Build history of the part. All positions in model axes, mm. Round coordinates to 2 decimals unless told otherwise and drop trailing zeros. Write each loop counter-clockwise with the first axis right and the second up, starting at its lowest first coordinate (ties: lowest second). Pieces come first, ordered by that corner, then holes. Notation, with made-up numbers: (11, 18.5) -> (55, 18.5) arc R22 ccw to (55, 54.5) -> close; hole circle Ø6 at (13, 1.5). An arc over 180 degrees is marked (long way). Answer in a Markdown table with one row per item. Add a question column.
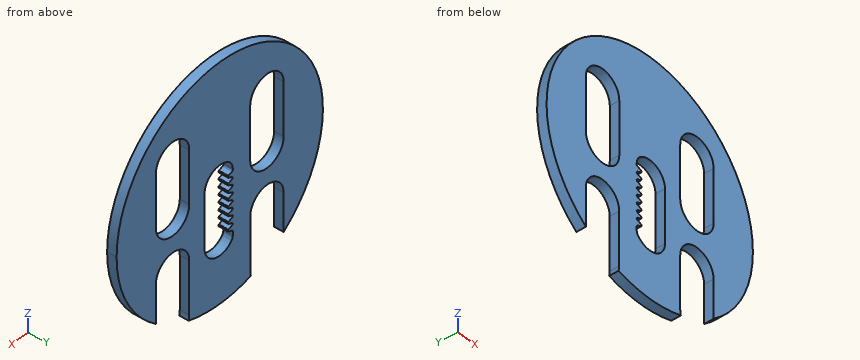
from build123d import *

# Parameters (mm, degrees)
BOSS_EXTRUDE1_DEPTH = 3.175
BOSS_EXTRUDE3_START = -3.175
BOSS_EXTRUDE3_DEPTH = 3.175


# Read off the part's stored shape, not the designer's step: Boss-Extrude3
with BuildPart() as part:
    # Sketch3 → Boss-Extrude1 (new body)
    with BuildSketch(Plane.XZ):
        with BuildLine():
            ThreePointArc((39.2557, 0), (-17.127226966, 35.322345321), (-24.310512242, -30.822215641))
            Line((-24.310512242, -30.822215641), (-24.310512242, -17.960512242))
            ThreePointArc((-24.310512242, -17.960512242), (-17.960512242, -11.610512242), (-11.610512242, -17.960512242))
            Line((-11.610512242, -17.960512242), (-11.610512242, -35.740512242))
            ThreePointArc((-11.610512242, -35.740512242), (-11.667849962, -36.591923676), (-11.838827653, -37.427959366))
            ThreePointArc((-11.838827653, -37.427959366), (0, -39.2557), (11.838827653, -37.427959366))
            ThreePointArc((11.838827653, -37.427959366), (11.667849962, -36.591923676), (11.610512242, -35.740512242))
            Line((11.610512242, -35.740512242), (11.610512242, -17.960512242))
            ThreePointArc((11.610512242, -17.960512242), (17.960512242, -11.610512242), (24.310512242, -17.960512242))
            Line((24.310512242, -17.960512242), (24.310512242, -30.822215641))
            ThreePointArc((24.310512242, -30.822215641), (35.322345321, -17.127226966), (39.2557, 0))
        make_face()
        with BuildLine():
            ThreePointArc((-5.8, 0), (0, 5.8), (5.8, 0))
            Line((5.8, 0), (5.8, -17.78))
            ThreePointArc((5.8, -17.78), (0, -23.58), (-5.8, -17.78))
            Line((-5.8, -17.78), (-5.8, 0))
        make_face(mode=Mode.SUBTRACT)
        with BuildLine():
            ThreePointArc((-11.590512242, 0.180512242), (-17.960512242, -6.189487758), (-24.330512242, 0.180512242))
            Line((-24.330512242, 0.180512242), (-24.330512242, 17.960512242))
            ThreePointArc((-24.330512242, 17.960512242), (-17.960512242, 24.330512242), (-11.590512242, 17.960512242))
            Line((-11.590512242, 17.960512242), (-11.590512242, 0.180512242))
        make_face(mode=Mode.SUBTRACT)
        with BuildLine():
            ThreePointArc((24.310512242, 0.180512242), (17.960512242, -6.169487758), (11.610512242, 0.180512242))
            Line((11.610512242, 0.180512242), (11.610512242, 17.960512242))
            ThreePointArc((11.610512242, 17.960512242), (17.960512242, 24.310512242), (24.310512242, 17.960512242))
            Line((24.310512242, 17.960512242), (24.310512242, 0.180512242))
        make_face(mode=Mode.SUBTRACT)
    extrude(amount=BOSS_EXTRUDE1_DEPTH)

    # Boss-Extrude3 outline → Boss-Extrude3 (add)
    with BuildSketch(Plane(origin=(0, 0, 0), x_dir=(1, 0, 0), z_dir=(0, 1, 0)).offset(BOSS_EXTRUDE3_START)):
        with BuildLine():
            Line((-4.952891864, -1.684975141), (-4.952891864, -1.246819584))
            ThreePointArc((-4.952891864, -1.246819584), (-4.879618202, -1.014425219), (-4.6863, -0.866086946))
            Line((-4.6863, -0.866086946), (-3.328347771, -0.371832755))
            ThreePointArc((-3.328347771, -0.371832755), (-3.253985597, -0.314772651), (-3.2258, -0.22537936))
            Line((-3.2258, -0.22537936), (-3.2258, 0.22537936))
            ThreePointArc((-3.2258, 0.22537936), (-3.253985597, 0.314772651), (-3.328347771, 0.371832755))
            Line((-3.328347771, 0.371832755), (-4.6863, 0.866086946))
            ThreePointArc((-4.6863, 0.866086946), (-4.952891864, 1.246819585), (-4.6863, 1.627552223))
            Line((-4.6863, 1.627552223), (-3.328347771, 2.121806414))
            ThreePointArc((-3.328347771, 2.121806414), (-3.253985597, 2.178866518), (-3.2258, 2.268259809))
            Line((-3.2258, 2.268259809), (-3.2258, 2.719018529))
            ThreePointArc((-3.2258, 2.719018529), (-3.253985597, 2.80841182), (-3.328347771, 2.865471924))
            Line((-3.328347771, 2.865471924), (-4.6863, 3.359726115))
            ThreePointArc((-4.6863, 3.359726115), (-4.952891864, 3.740458754), (-4.6863, 4.121191392))
            Line((-4.6863, 4.121191392), (-3.328347771, 4.615445582))
            ThreePointArc((-3.328347771, 4.615445582), (-3.253985597, 4.672505686), (-3.2258, 4.761898978))
            Line((-3.2258, 4.761898978), (-3.2258, 5.212657697))
            ThreePointArc((-3.2258, 5.212657697), (-3.253985597, 5.302050989), (-3.328347771, 5.359111093))
            Line((-3.328347771, 5.359111093), (-4.6863, 5.853365283))
            ThreePointArc((-4.6863, 5.853365283), (-4.952891864, 6.234097921), (-4.6863, 6.61483056))
            Line((-4.6863, 6.61483056), (-3.328347771, 7.109084751))
            ThreePointArc((-3.328347771, 7.109084751), (-3.253985597, 7.166144855), (-3.2258, 7.255538147))
            Line((-3.2258, 7.255538147), (-3.2258, 7.706296866))
            ThreePointArc((-3.2258, 7.706296866), (-3.253985597, 7.795690157), (-3.328347771, 7.852750261))
            Line((-3.328347771, 7.852750261), (-4.6863, 8.347004452))
            ThreePointArc((-4.6863, 8.347004452), (-4.952891864, 8.72773709), (-4.6863, 9.108469729))
            Line((-4.6863, 9.108469729), (-3.328347771, 9.60272392))
            ThreePointArc((-3.328347771, 9.60272392), (-3.253985597, 9.659784024), (-3.2258, 9.749177315))
            Line((-3.2258, 9.749177315), (-3.2258, 10.199936035))
            ThreePointArc((-3.2258, 10.199936035), (-3.253985597, 10.289329326), (-3.328347771, 10.34638943))
            Line((-3.328347771, 10.34638943), (-4.6863, 10.840643621))
            ThreePointArc((-4.6863, 10.840643621), (-4.952891864, 11.221376259), (-4.6863, 11.602108898))
            Line((-4.6863, 11.602108898), (-3.328347771, 12.096363089))
            ThreePointArc((-3.328347771, 12.096363089), (-3.253985597, 12.153423193), (-3.2258, 12.242816484))
            Line((-3.2258, 12.242816484), (-3.2258, 12.693575204))
            ThreePointArc((-3.2258, 12.693575204), (-3.253985597, 12.782968495), (-3.328347771, 12.840028599))
            Line((-3.328347771, 12.840028599), (-4.6863, 13.33428279))
            ThreePointArc((-4.6863, 13.33428279), (-4.952891864, 13.715015428), (-4.6863, 14.095748067))
            Line((-4.6863, 14.095748067), (-3.328347771, 14.590002258))
            ThreePointArc((-3.328347771, 14.590002258), (-3.253985597, 14.647062362), (-3.2258, 14.736455653))
            Line((-3.2258, 14.736455653), (-3.2258, 15.187214372))
            ThreePointArc((-3.2258, 15.187214372), (-3.253985597, 15.276607664), (-3.328347771, 15.333667768))
            Line((-3.328347771, 15.333667768), (-4.6863, 15.827921959))
            ThreePointArc((-4.6863, 15.827921959), (-4.952891864, 16.208654598), (-4.6863, 16.589387236))
            Line((-4.6863, 16.589387236), (-3.328347771, 17.083641426))
            ThreePointArc((-3.328347771, 17.083641426), (-3.253985597, 17.14070153), (-3.2258, 17.230094822))
            Line((-3.2258, 17.230094822), (-3.2258, 17.680853541))
            ThreePointArc((-3.2258, 17.680853541), (-3.253985597, 17.770246833), (-3.328347771, 17.827306937))
            Line((-3.328347771, 17.827306937), (-4.6863, 18.321561127))
            ThreePointArc((-4.6863, 18.321561127), (-4.879618202, 18.469899401), (-4.952891864, 18.702293766))
            Line((-4.952891864, 18.702293766), (-4.952891864, 20.205203806))
            ThreePointArc((-4.952891864, 20.205203806), (-4.846345509, 20.833344029), (-4.538625549, 21.391215602))
            ThreePointArc((-4.538625549, 21.391215602), (-5.475583448, 19.692586183), (-5.8, 17.78))
            Line((-5.8, 17.78), (-5.8, 0))
            ThreePointArc((-5.8, 0), (-5.240594871, -2.485189209), (-3.670287792, -4.490989593))
            Line((-3.670287792, -4.490989593), (-3.66100885, -4.494366852))
            ThreePointArc((-3.66100885, -4.494366852), (-4.614444615, -3.231070506), (-4.952891864, -1.684975141))
        make_face()
    extrude(amount=BOSS_EXTRUDE3_DEPTH)


solid = part.part
(1) Saw through at D-D (z = 20.5). List the corners of the cut face in (x, y) (3 decimals), plus the area to 3 significant figures.
(2) Drop flat-ended pins along their axis: P1, Ø1, axis at y = -2, z = -22, coming from the +X side; P2, Ø1.6, axis at y = -2, z = -22.5, coming from the -X side; P3, Ø1.7, axis at y = -1, z = -20, coming from the +X side. Give the stop position or say it passes through.
(3) Saw through at C-C (y = -0.5). Count the separate pieces of the cut face and the enclosed holes in it, plus the area to 3 significant figures.
(4) Probe line 1 along X through (y, z) = (-0.05, 3); line 2 along X through (y, z) = (-1, 23.5); line 3 along X through (y, z) = (-2.6, 13). List the from-to ranges inside material, lowest first.
(5) Saw through at B-B (z = 9.5). List the corners of the cut face in (x, y) (3 decimals), plus the area to 3 significant figures.
(6) Saw through at A-A (x = 0). List the corners of the cut face in (y, z) (3 decimals).
Answer sheet:
| question | item | result |
|---|---|---|
| 1 | outline | (-33.478, -3.175) -> (-23.802, -3.175) -> (-23.802, 0) -> (-33.478, 0) -> close; (-12.119, -3.175) -> (12.14, -3.175) -> (12.14, 0) -> (-12.119, 0) -> close; (23.781, -3.175) -> (33.478, -3.175) -> (33.478, 0) -> (23.781, 0) -> close |
| 1 | area | 139 mm² |
| 2 | P1 | stops at x = 32.84 |
| 2 | P2 | stops at x = -32.71 |
| 2 | P3 | stops at x = 34.27 |
| 3 | separate pieces | 1 |
| 3 | enclosed holes | 3 |
| 3 | area | 3,310 mm² |
| 4 | line 1 | x = -39.14 to -24.33, -11.59 to -4.71, 4.96 to 11.61, 24.31 to 39.14 |
| 4 | line 2 | x = -31.44 to -21.11, -14.82 to 14.86, 21.06 to 31.44 |
| 4 | line 3 | x = -37.04 to -24.33, -11.59 to 11.61, 24.31 to 37.04 |
| 5 | outline | (-38.089, -3.175) -> (-24.331, -3.175) -> (-24.331, 0) -> (-38.089, 0) -> close; (-11.591, -3.175) -> (11.611, -3.175) -> (11.611, 0) -> (-11.591, 0) -> close; (24.311, -3.175) -> (38.089, -3.175) -> (38.089, 0) -> (24.311, 0) -> close |
| 5 | area | 161 mm² |
| 6 | outline | (-3.175, -39.256) -> (0, -39.256) -> (0, -23.58) -> (-3.175, -23.58) -> close; (-3.175, 5.8) -> (0, 5.8) -> (0, 39.256) -> (-3.175, 39.256) -> close |
